from build123d import *

# Parameters (mm, degrees)
F1_DEPTH = 2
F2_D     = 4.4
F2_DEPTH = 5
F2_TIP   = 1.3218933619


# Not quite as in the source:
# - ends of sketch curves that miss each other by under 0.0002 mm in the source are joined


with BuildPart() as f1:
    # F0 (on Top) → F1 (new body)
    with BuildSketch(Plane.XY):
        with BuildLine():
            Line((24, 0), (0, 0))
            Line((0, 0), (0, -31.5))
            Line((0, -31.5), (12, -31.5))
            ThreePointArc((12, -31.5), (12.8786796564, -29.3786796564), (15, -28.5))
            Line((15, -28.5), (24, -28.5))
            Line((24, -28.5), (24, -26.4939))
            Line((24, -26.4939), (15.0018, -26.4939))
            ThreePointArc((15.0018, -26.4939), (13.5919063065, -25.9124202759), (13.001837209, -24.506099773))
            Line((13.001837209, -24.506099773), (13.0018, -24.4939))
            ThreePointArc((13.0018, -24.4939), (13.5919063065, -23.0875797241), (15.0018, -22.5061))
            Line((15.0018, -22.5061), (24, -22.5061))
            Line((24, -22.5061), (24, 0))
        make_face()
        with BuildLine():
            Line((48, 0), (24, 0))
            Line((24, 0), (24, -22.5061))
            Line((24, -22.5061), (32.9982, -22.5061))
            ThreePointArc((32.9982, -22.5061), (34.4080936935, -23.0875797241), (34.998162791, -24.493900227))
            Line((34.998162791, -24.493900227), (34.9982, -24.5061))
            ThreePointArc((34.9982, -24.5061), (34.4080936935, -25.9124202759), (32.9982, -26.4939))
            Line((32.9982, -26.4939), (24, -26.4939))
            Line((24, -26.4939), (24, -28.5))
            Line((24, -28.5), (33, -28.5))
            ThreePointArc((33, -28.5), (35.1213203436, -29.3786796564), (36, -31.5))
            Line((36, -31.5), (48, -31.5))
            Line((48, -31.5), (48, 0))
        make_face()
        with BuildLine():
            Line((12, -31.5), (0, -31.5))
            Line((0, -31.5), (0, -63))
            Line((0, -63), (24, -63))
            Line((24, -63), (24, -40.5224670172))
            Line((24, -40.5224670172), (15, -40.5224670172))
            ThreePointArc((15, -40.5224670172), (13.5857864376, -39.9366805795), (13, -38.5224670172))
            ThreePointArc((13, -38.5224670172), (13.5857864376, -37.1082534548), (15, -36.5224670172))
            Line((15, -36.5224670172), (24, -36.5224670172))
            Line((24, -36.5224670172), (24, -34.5))
            Line((24, -34.5), (15, -34.5))
            ThreePointArc((15, -34.5), (12.8786796564, -33.6213203436), (12, -31.5))
        make_face()
        with BuildLine():
            Line((48, -63), (48, -31.5))
            Line((48, -31.5), (36, -31.5))
            ThreePointArc((36, -31.5), (35.1213203436, -33.6213203436), (33, -34.5))
            Line((33, -34.5), (24, -34.5))
            Line((24, -34.5), (24, -36.5224670172))
            Line((24, -36.5224670172), (33, -36.5224670172))
            ThreePointArc((33, -36.5224670172), (34.4142135624, -37.1082534548), (35, -38.5224670172))
            ThreePointArc((35, -38.5224670172), (34.4142135624, -39.9366805795), (33, -40.5224670172))
            Line((33, -40.5224670172), (24, -40.5224670172))
            Line((24, -40.5224670172), (24, -63))
            Line((24, -63), (48, -63))
        make_face()
    extrude(amount=F1_DEPTH)

    # F2
    with Locations(Plane(origin=(0, 0, 0), x_dir=(1, 0, 0), z_dir=(0, 0, -1))):
        with Locations((5, 5), (43, 5), (43, 58), (5, 58)):
            Hole(F2_D / 2, depth=F2_DEPTH)
            with Locations((0, 0, -(F2_DEPTH + F2_TIP / 2))):  # 118° drill point
                Cone(0, F2_D / 2, F2_TIP, mode=Mode.SUBTRACT)


solid = f1.part
The model under review builds one solid part; all positions refer to its coordinate system, in mm. A direction names the side the tool comes from. Coordinates: 2 decimals unless noted, no trailing zeros. Loops run counter-clockwise (first coordinate to the right, second up) from the corner with the lowest first, then second, coordinate; pieces in that order, holes last. Notation, with made-up numbers: M 8,2.25 L 39,2.25 A26 ccw 39,26.25 Z; hole C 6.25,45.25 d1. An arc over 180 degrees is marked long. Put each result on its own line as item: value. Start each with the question number.
Q1. Add section B-B (z = 1.5). Count the separate pieces of the cut face and the enclosed holes in it, and give its area (3 significant figures).
Q2. Add section A-A (x = 5). Write out the cut boundary in (y, z).
Q3. For faces 5 (the flat face through (48, -32, 1)), 6 (the cylindrical face through (34.42, -25.9, 0.99)), list the 3-axis set-ups (+Z, -Z, +X, -X, +Y, -Y) from which the entire face can be reached by the end or side of a thin tool; tool diameter is ignored.
Q4. The part is to be moulded in two halves that separate along X. For faces 1 (the flat face through (0, -31, 1)), 2 (the flat face through (24, -40.522, 1)), 3 (the flat face through (24, -17, 0)), 4 (the flat face through (24, -22.506, 1)), say which applies: +X half, -X half, draft (parallel to the pull), parting line (faces both ways), or undercut.
Q5. Add section D-D (x = 26). Write out the cut boundary in (y, z), and give its area (3 significant figures).
Q6. Wall thickness on line 1 (Y direction, x = 43, z = 1.2); line 2 (Y direction, x = 17, z = 1.6); line 3 (X direction, y = -58, z = 1.4): over which ranges is each line inside the solid? List them lowest first.
Q7. Add section C-C (y = -5). Write out the cut boundary in (x, z).
Q8. Clearance check with a flat-ended pin moving along its axis: pin 1 (4 mm diameter, centred on x = 5, y = -5, fed in from -Z). State where the tip first meets the part, or that it passes through.
Answers:
1. separate pieces: 1
1. enclosed holes: 7
1. area: 2,660 mm^2
2. outline: M -63,0 L -60.2,0 L -60.2,2 L -63,2 Z; M -55.8,0 L -7.2,0 L -7.2,2 L -55.8,2 Z; M -2.8,0 L 0,0 L 0,2 L -2.8,2 Z
3. face 5: +Z, -Z, +X, +Y, -Y
3. face 6: +Z, -Z
4. face 1: -X half
4. face 2: undercut
4. face 3: draft
4. face 4: undercut
5. outline: M -63,0 L -40.52,0 L -40.52,2 L -63,2 Z; M -36.52,0 L -34.5,0 L -34.5,2 L -36.52,2 Z; M -28.5,0 L -26.49,0 L -26.49,2 L -28.5,2 Z; M -22.51,0 L 0,0 L 0,2 L -22.51,2 Z
5. area: 98.0 mm^2
6. line 1: y = -63 to -60.2, -55.8 to -7.2, -2.8 to 0
6. line 2: y = -63 to -40.52, -36.52 to -34.5, -28.5 to -26.49, -22.51 to 0
6. line 3: x = 0 to 2.8, 7.2 to 40.8, 45.2 to 48
7. outline: M 0,0 L 2.8,0 L 2.8,2 L 0,2 Z; M 7.2,0 L 40.8,0 L 40.8,2 L 7.2,2 Z; M 45.2,0 L 48,0 L 48,2 L 45.2,2 Z
8. pin 1: passes through
